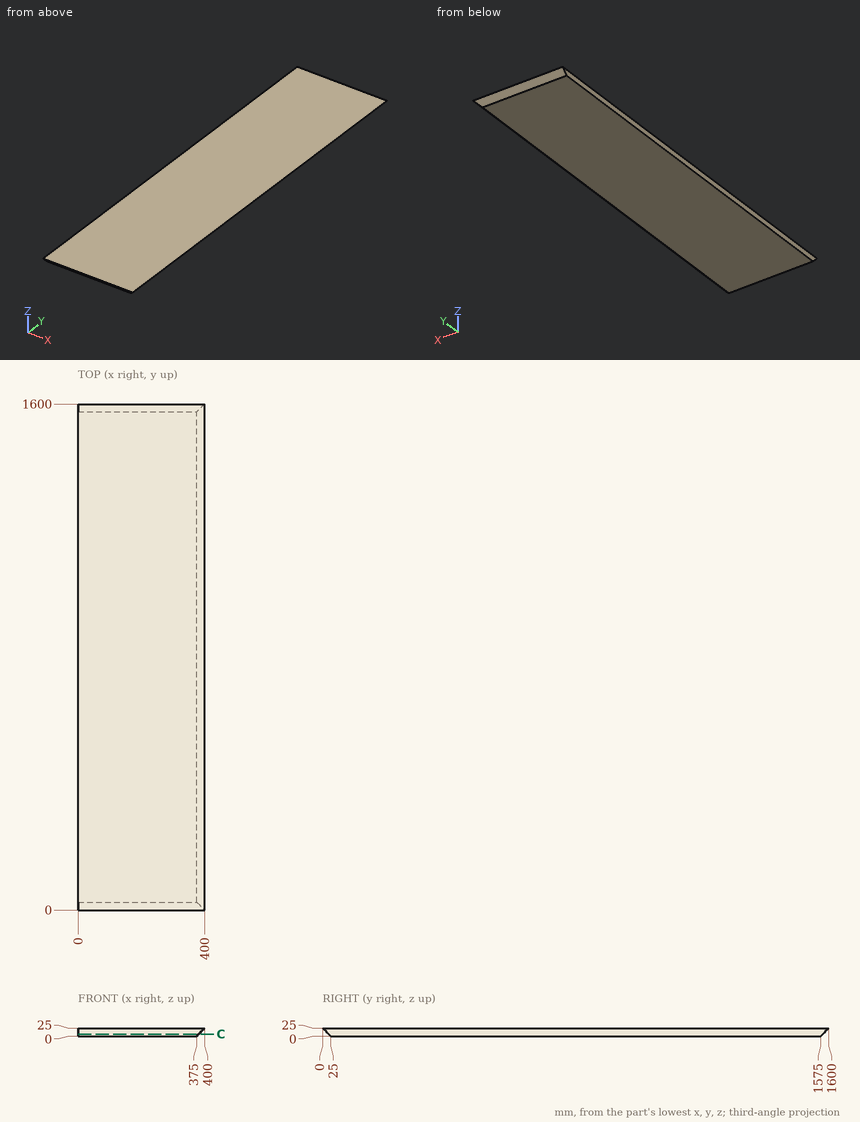
Here's the drawing with two shaded views (mm, measured from the low corner). I have some questions. Give positions to 0.01 mm unless a question says otherwise; leave off trailing zeros. Order: outer loops, then holes, each group sorted by start corner. A loop starts at its lowest first (then second) coordinate and runs counter-clockwise, first axis right, second up. Notation, with made-up numbers: M 9,25 L 23,25 A8 cw 23,39 Z; hole C 61.25,37.5 d1. An arc over 180 degrees is marked long. One line per item, written item: value.
1) Please list where these lines run through material, in increasing order: line 1 along X through (y, z) = (1302, 7.5); line 2 along X through (y, z) = (513.5, 21.5); line 3 along Y through (x, z) = (272, 18.75).
Answer sheet:
line 1: x = 0 to 382.5
line 2: x = 0 to 396.5
line 3: y = 6.25 to 1593.75
2) For P1, Ø5, axis at x = 157.5, z = 6, coming from the -Y side; P2, Ø6, axis at x = 318, z = 19, coming from the -Y side; P3, Ø6, axis at x = 88.5, z = 15, coming from the -Y side, each with a flat end and sliding along its axis, tell me the tip position at first contact or that it passes through.
Answer sheet:
P1: stops at y = 16.5
P2: stops at y = 3
P3: stops at y = 7
3) I want a section at C-C, the plane z = 5.75. List the corners of the cut face in (x, y) for me, plus the area to 3 significant figures.
Answer sheet:
outline: M 0,19.25 L 380.75,19.25 L 380.75,1580.75 L 0,1580.75 Z
area: 595,000 mm^2
